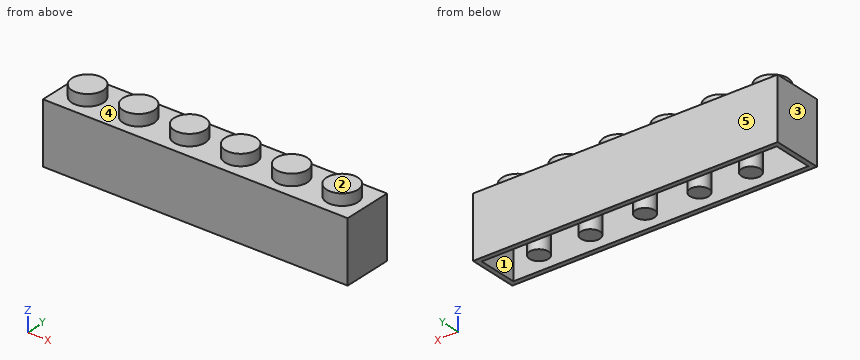
```python
from build123d import *

# Parameters (mm, degrees)
F0_W      = 47.7774
F0_H      = 7.8232
F1_DEPTH  = 4.78155
F2_R      = 2.4511
F8_DEPTH  = 1.778
F3_R      = 2.4511
F9_DEPTH  = 1.778
F4_R      = 2.4511
F10_DEPTH = 1.778
F5_R      = 2.4511
F11_DEPTH = 1.778
F6_R      = 2.4511
F12_DEPTH = 1.778
F7_R      = 2.4511
F13_DEPTH = 1.778
F14_W     = 46.2534
F14_H     = 6.2992
F20_DEPTH = 8.3312
F15_R     = 1.4859
F21_DEPTH = 8.3312
F16_R     = 1.4859
F22_DEPTH = 8.3312
F17_R     = 1.4859
F23_DEPTH = 8.3312
F19_R     = 1.4859
F24_DEPTH = 8.3312
F18_R     = 1.4859
F25_DEPTH = 8.3312


with BuildPart() as f1:
    # F0 (on Top) → F1 (new body, symmetric)
    with BuildSketch(Plane.XY):
        Rectangle(F0_W, F0_H)
    extrude(amount=F1_DEPTH, both=True)

    # F2 (on face) → F8 (join)
    with BuildSketch(Plane.XY.offset(4.78155)):
        with Locations((-19.9644, -0.0127)):
            Circle(F2_R)
    extrude(amount=F8_DEPTH)

    # F3 (on face) → F9 (join)
    with BuildSketch(Plane.XY.offset(4.78155)):
        with Locations((-11.9634, -0.0127)):
            Circle(F3_R)
    extrude(amount=F9_DEPTH)

    # F4 (on face) → F10 (join)
    with BuildSketch(Plane.XY.offset(4.78155)):
        with Locations((-3.9624, -0.0127)):
            Circle(F4_R)
    extrude(amount=F10_DEPTH)

    # F5 (on face) → F11 (join)
    with BuildSketch(Plane.XY.offset(4.78155)):
        with Locations((4.0386, -0.0127)):
            Circle(F5_R)
    extrude(amount=F11_DEPTH)

    # F6 (on face) → F12 (join)
    with BuildSketch(Plane.XY.offset(4.78155)):
        with Locations((12.0396, -0.0127)):
            Circle(F6_R)
    extrude(amount=F12_DEPTH)

    # F7 (on face) → F13 (join)
    with BuildSketch(Plane.XY.offset(4.78155)):
        with Locations((19.9644, -0.0127)):
            Circle(F7_R)
    extrude(amount=F13_DEPTH)

    # F14 (on face) → F20 (cut)
    with BuildSketch(Plane(origin=(0, 0, -4.78155), x_dir=(1, 0, 0), z_dir=(0, 0, -1))):
        Rectangle(F14_W, F14_H)
    extrude(amount=-F20_DEPTH, mode=Mode.SUBTRACT)

    # F15 (on face) → F21 (join)
    with BuildSketch(Plane(origin=(0, 0, -4.78155), x_dir=(1, 0, 0), z_dir=(0, 0, -1))):
        with Locations((-16.6116, 0)):
            Circle(F15_R)
    extrude(amount=-F21_DEPTH)

    # F16 (on face) → F22 (join)
    with BuildSketch(Plane(origin=(0, 0, -4.78155), x_dir=(1, 0, 0), z_dir=(0, 0, -1))):
        with Locations((-8.5344, 0)):
            Circle(F16_R)
    extrude(amount=-F22_DEPTH)

    # F17 (on face) → F23 (join)
    with BuildSketch(Plane(origin=(0, 0, -4.78155), x_dir=(1, 0, 0), z_dir=(0, 0, -1))):
        Circle(F17_R)
    extrude(amount=-F23_DEPTH)

    # F19 (on face) → F24 (join)
    with BuildSketch(Plane(origin=(0, 0, -4.78155), x_dir=(1, 0, 0), z_dir=(0, 0, -1))):
        with Locations((8.5598, 0)):
            Circle(F19_R)
    extrude(amount=-F24_DEPTH)

    # F18 (on face) → F25 (join)
    with BuildSketch(Plane(origin=(0, 0, -4.78155), x_dir=(1, 0, 0), z_dir=(0, 0, -1))):
        with Locations((16.6116, 0)):
            Circle(F18_R)
    extrude(amount=-F25_DEPTH)


solid = f1.part
```
Source: CAD feature listing. Evaluate the final solid. Frame: model axes, mm. Face numbers are marked on the shaded views. A direction names the side the tool comes from. Coordinates: 2 decimals unless noted, no trailing zeros. Write each loop counter-clockwise with the first axis right and the second up, starting at its lowest first coordinate (ties: lowest second). Pieces come first, ordered by that corner, then holes. Notation, with made-up numbers: M -2,38 L 39,38 A34 cw 39,72 Z; hole C 8.25,45 d8. An arc over 180 degrees is marked long. Answer as a JSON object with one key per item and string values.
1. Cut plane D-D on z = 5.25. Output: boundary loops of the cut face in (x, y), plus the area to 3 significant figures.
Evaluation:
{"outline": "C -19.96,-0.01 d4.9; C -11.96,-0.01 d4.9; C -3.96,-0.01 d4.9; C 4.04,-0.01 d4.9; C 12.04,-0.01 d4.9; C 19.96,-0.01 d4.9", "area": "113 mm^2"}
2. Ray query, L1, parallel to X at y = 2.75, z = -2; L2, parallel to Y at x = -9.5, z = -3.75; L3, parallel to Y at x = 10.5, z = 0.5. Return the intervals inside material, ascending.
Evaluation:
{"L1": "-23.89 to -23.13, 23.13 to 23.89", "L2": "-3.91 to -3.15, -1.13 to 1.13, 3.15 to 3.91", "L3": "-3.91 to -3.15, 3.15 to 3.91"}
3. Access query for the marked faces 1 and 2. Directions: +Z, -Z, +X, -X, +Y, -Y. A direction counts if a zero-diameter tool reaches every point of the face in a straight line with its end or side. Return the directions, or none.
Evaluation:
{"face 1": "-Z", "face 2": "+Z, +X, -X, +Y, -Y"}
4. Cut plane B-B on x = 0. Output: boundary loops of the cut face in (y, z).
Evaluation:
{"outline": "M -3.91,-4.78 L -3.15,-4.78 L -3.15,3.55 L -1.49,3.55 L -1.49,-4.78 L 1.49,-4.78 L 1.49,3.55 L 3.15,3.55 L 3.15,-4.78 L 3.91,-4.78 L 3.91,4.78 L -3.91,4.78 Z"}
5. Contact query for a flat-ended pin moving along its axis: P1, Ø1.5, axis at x = 8, y = 2, coming from the +Z side. Output: stop coordinate, or through.
Evaluation:
{"P1": "z = 4.78"}
6. Cut plane A-A on z = 2.5. Output: boundary loops of the cut face in (x, y).
Evaluation:
{"outline": "M -23.89,-3.91 L 23.89,-3.91 L 23.89,3.91 L -23.89,3.91 Z; C -16.61,0 d2.97; C -8.53,0 d2.97; C 0,0 d2.97; C 8.56,0 d2.97; C 16.61,0 d2.97; hole M -23.13,-3.15 L 23.13,-3.15 L 23.13,3.15 L -23.13,3.15 Z"}
7. Draft query along X for the marked faces 3, 4 and 5. Return one class per face: released by +X, released by -X, zero draft, split by the parting line, or undercut.
Evaluation:
{"face 3": "released by -X", "face 4": "undercut", "face 5": "zero draft"}
